The model under review builds one solid part; all positions refer to its coordinate system, in mm. A direction names the side the tool comes from. Coordinates: 2 decimals unless noted, no trailing zeros. Order: outer loops, then holes, each group sorted by start corner. A loop starts at its lowest first (then second) coordinate and runs counter-clockwise, first axis right, second up. Notation, with made-up numbers: (42.25, 52) -> (69.25, 52) arc R17 cw to (69.25, 59) -> close; hole circle Ø10 at (50, -11). An arc over 180 degrees is marked (long way). Put each result on its own line as item: value.
from build123d import *

# Parameters (mm, degrees)
SKETCH1_W                      = 25.4
SKETCH1_H                      = 50.8
BOSS_EXTRUDE1_DEPTH            = 30
SKETCH2_W                      = 25.4
SKETCH2_H                      = 25
CUT_EXTRUDE1_DEPTH             = 12
M12_CLEARANCE_HOLE1_D          = 12.5
M5X0_8_TAPPED_HOLE1_AT_2_COUNT = 2
M5X0_8_TAPPED_HOLE1_AT_2_PITCH = 30
CHAMFER1_0_5_MM_SIZE           = 0.5


with BuildPart() as part:
    # Sketch1 → Boss-Extrude1 (new body)
    with BuildSketch(Plane.XY):
        Rectangle(SKETCH1_W, SKETCH1_H)
    extrude(amount=BOSS_EXTRUDE1_DEPTH)

    # Sketch2 → Cut-Extrude1 (cut)
    with BuildSketch(Plane.XY):
        Rectangle(SKETCH2_W, SKETCH2_H)
    extrude(amount=CUT_EXTRUDE1_DEPTH, mode=Mode.SUBTRACT)

    # M12 Clearance Hole1 (through all)
    with Locations(Plane(origin=(0, 0, 12), x_dir=(-1, 0, 0), z_dir=(0, 0, -1))):
        with Locations((0, 0)):
            Hole(M12_CLEARANCE_HOLE1_D / 2)

    # Sketch11 → M5x0.8 Tapped Hole1 (revolve, cut)
    with BuildSketch(Plane(origin=(12.7, 15, 21), x_dir=(0, 0, -1), z_dir=(0, 1, 0))):
        Polygon((0, 0), (0, 12), (2.1, 10.7381927), (2.1, 0), align=None)
    m5x0_8_tapped_hole1 = revolve(axis=Axis((19.05, 15, 21), (-1, 0, 0)), mode=Mode.SUBTRACT)

    # M5x0.8 Tapped Hole1 at 2: M5x0.8 Tapped Hole1 ×2
    with Locations(*[(0, -i * M5X0_8_TAPPED_HOLE1_AT_2_PITCH, 0) for i in range(1, M5X0_8_TAPPED_HOLE1_AT_2_COUNT)]):
        add(m5x0_8_tapped_hole1, mode=Mode.SUBTRACT)

    # Mirror1: M5x0.8 Tapped Hole1 across plane
    add(m5x0_8_tapped_hole1.mirror(Plane(origin=(0, 0, 0), x_dir=(0, 0, 1), z_dir=(1, 0, 0))), mode=Mode.SUBTRACT)

    # Mirror1 copy 1 sketch → Mirror1 copy 1 (revolve, cut)
    with BuildSketch(Plane(origin=(-12.7, -15, 21), x_dir=(0, 0, -1), z_dir=(0, 1, 0))):
        Polygon((0, 0), (0, -12), (2.1, -10.7381927), (2.1, 0), align=None)
    revolve(axis=Axis((-19.05, -15, 21), (-1, 0, 0)), mode=Mode.SUBTRACT)

    # Chamfer1 0.5 mm
    chamfer1_0_5_mm_edges = [part.edges().sort_by_distance(p)[0] for p in [
        (-6.25, 0, 12),
        (-6.25, 0, 30),
        (12.7, -15, 23.1),
        (12.7, 15, 23.1),
        (-12.7, -15, 23.1),
        (-12.7, 15, 23.1),
    ]]
    chamfer(chamfer1_0_5_mm_edges, length=CHAMFER1_0_5_MM_SIZE)


solid = part.part
Item 1: Consider section C-C on y = 0. Write out the cut boundary in (x, z).
Answers below:
outline: (-12.7, 12) -> (-6.75, 12) -> (-6.25, 12.5) -> (-6.25, 29.5) -> (-6.75, 30) -> (-12.7, 30) -> close; (6.25, 12.5) -> (6.75, 12) -> (12.7, 12) -> (12.7, 30) -> (6.75, 30) -> (6.25, 29.5) -> close
Item 2: For faces 1 (the flat face through (5, 6, 12)), 2 (the cylindrical face through (7.15, -12.95, 21.46)), 3 (the cylindrical face through (-7.153, -17.082, 21.273)), list the 3-axis set-ups (+Z, -Z, +X, -X, +Y, -Y) from which the entire face can be reached by the end or side of a thin tool; tool diameter is ignored.
Answers below:
face 1: -Z, +X, -X
face 2: +X
face 3: -X
Item 3: Consider section A-A on z = 3. Write out the cut boundary in (x, y), and give its area (3 significant figures).
Answers below:
outline: (-12.7, -25.4) -> (12.7, -25.4) -> (12.7, -12.5) -> (-12.7, -12.5) -> close; (-12.7, 12.5) -> (12.7, 12.5) -> (12.7, 25.4) -> (-12.7, 25.4) -> close
area: 655 mm^2
Item 4: For pin 1 Ø3.5 at (y, z) = (-15, 21) entering from +X; pin 2 Ø5 at (y, z) = (-15, 21) entering from -X; pin 3 Ø4 at (y, z) = (15, 21) entering from -X, all flat-tipped, find the tip position at first contact; note any pin that passes through.
Answers below:
pin 1: x = 1.75
pin 2: x = -12.6
pin 3: x = -1.9
Item 5: Consider section D-D on x = -11. Write out the cut boundary in (y, z).
Answers below:
outline: (-25.4, 0) -> (-12.5, 0) -> (-12.5, 12) -> (12.5, 12) -> (12.5, 0) -> (25.4, 0) -> (25.4, 30) -> (-25.4, 30) -> close; hole circle Ø4.2 at (-15, 21); hole circle Ø4.2 at (15, 21)
Item 6: Consider section B-B on x = 0. Write out the cut boundary in (y, z).
Answers below:
outline: (-25.4, 0) -> (-12.5, 0) -> (-12.5, 12) -> (-6.75, 12) -> (-6.25, 12.5) -> (-6.25, 29.5) -> (-6.75, 30) -> (-25.4, 30) -> close; (6.25, 12.5) -> (6.75, 12) -> (12.5, 12) -> (12.5, 0) -> (25.4, 0) -> (25.4, 30) -> (6.75, 30) -> (6.25, 29.5) -> close
Item 7: Mouldability with a two-part tool opening along X and no side actions: class faces 4 (the conical face through (-0.919, 14.984, 21.364)), 5 (the cylindrical face through (7.15, 17.05, 21.46)), 6 (the flat face through (12.7, 0, 18)), 7 (the cylindrical face through (5.96, 1.88, 21.12)) as +X half, -X half, draft (parallel to the pull), parting line (faces both ways), or undercut.
Answers below:
face 4: -X half
face 5: draft
face 6: +X half
face 7: undercut
Item 8: For line 1 (Y direction, x = 6.5, z = 21); line 2 (Y direction, x = 2.75, z = 8.75); line 3 (Z direction, x = 4.5, y = -15), list the stretches that pass through material, from the lowest coordinate up. Write a range as from..to.
Answers below:
line 1: -25.4..-17.1, -12.9..12.9, 17.1..25.4
line 2: -25.4..-12.5, 12.5..25.4
line 3: 0..18.9, 23.1..30
